Can you work these out from the drawing? Everything is in mm from the part's minimum corner. A direction names the side the tool comes from. Give positions to 0.01 mm unless a question says otherwise; leave off trailing zeros. Write each loop counter-clockwise with the first axis right and the second up, starting at its lowest first coordinate (ties: lowest second). Pieces come first, ordered by that corner, then holes. Notation, with made-up numbers: (59, 7.25) - (76, 7.25) arc R22 cw to (76, 35.25) - close; hole circle Ø6 at (7, -5.5). An arc over 180 degrees is marked (long way). Use a Markdown table: item, result.
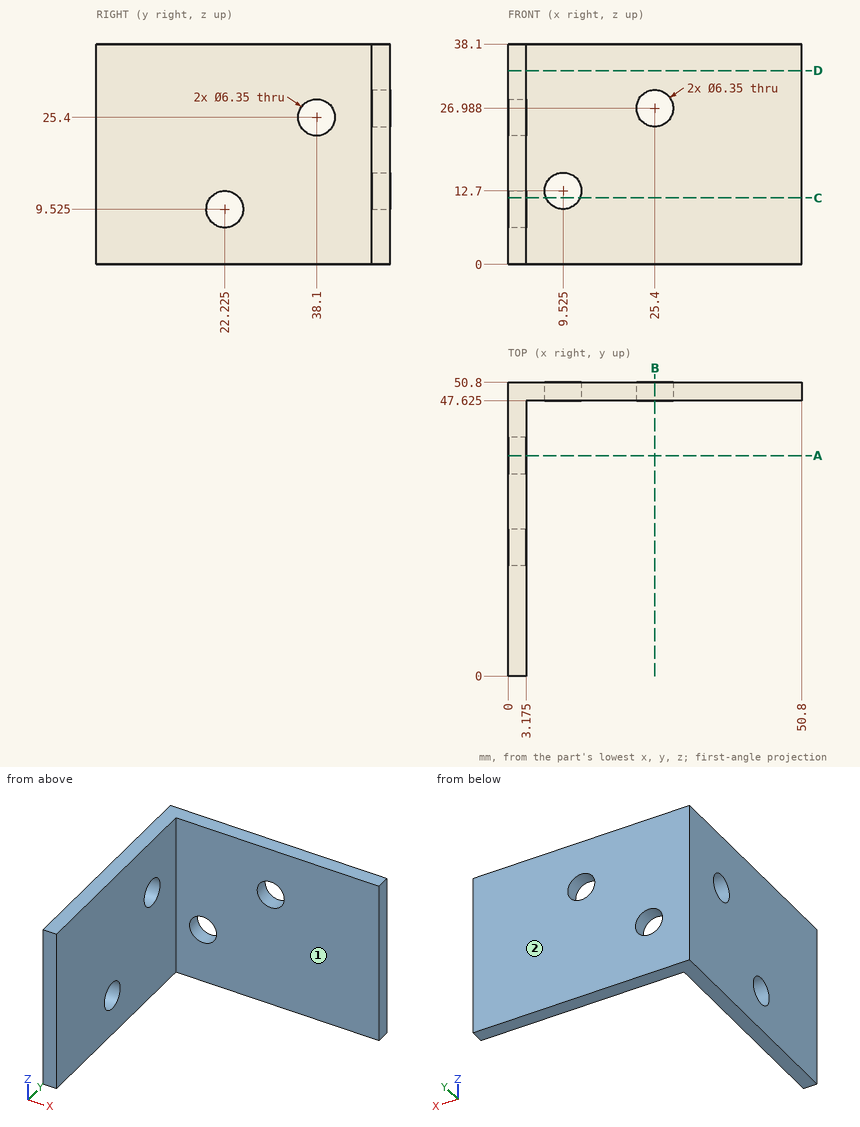
Item 1: If we section it at C-C, the plane z = 11.5: Write out the boundary of the cut face in (x, y) (1 decimal).
Values:
| item | result |
|---|---|
| outline | (0, 0) - (3.2, 0) - (3.2, 19.7) - (0, 19.7) - close; (0, 24.7) - (3.2, 24.7) - (3.2, 47.6) - (6.6, 47.6) - (6.6, 50.8) - (0, 50.8) - close; (12.5, 47.6) - (50.8, 47.6) - (50.8, 50.8) - (12.5, 50.8) - close |
Item 2: If we section it at B-B, the plane x = 25.4: Write out the boundary of the cut face in (y, z) (1 decimal).
Values:
| item | result |
|---|---|
| outline | (47.6, 0) - (50.8, 0) - (50.8, 23.8) - (47.6, 23.8) - close; (47.6, 30.2) - (50.8, 30.2) - (50.8, 38.1) - (47.6, 38.1) - close |
Item 3: If we section it at A-A, the plane y = 38.1: Write out the boundary of the cut face in (x, z) (1 decimal).
Values:
| item | result |
|---|---|
| outline | (0, 0) - (3.2, 0) - (3.2, 22.2) - (0, 22.2) - close; (0, 28.6) - (3.2, 28.6) - (3.2, 38.1) - (0, 38.1) - close |
Item 4: For the marked faces 1 and 2, which set-ups out of +Z, -Z, +X, -X, +Y, -Y let a thin tool reach every point of the face, with its end or its side?
Values:
| item | result |
|---|---|
| face 1 | +Z, -Z, +X, -Y |
| face 2 | +Z, -Z, +X, -X, +Y |
Item 5: I need wall thicknesses on line 1 along Z through (x, y) = (25.4, 49.65); line 2 along Y through (x, z) = (36.5, 24) (1 decimal); line 3 along X through (y, z) = (48.7, 12.7). Which ranges of each line are inside material? Lowest first, please. Write a range as [from, to].
Values:
| item | result |
|---|---|
| line 1 | z = [0, 23.81], [30.16, 38.1] |
| line 2 | y = [47.6, 50.8] |
| line 3 | x = [0, 6.35], [12.7, 50.8] |
Item 6: If we section it at D-D, the plane z = 33.5: Write out the boundary of the cut face in (x, y) (1 decimal).
Values:
| item | result |
|---|---|
| outline | (0, 0) - (3.2, 0) - (3.2, 47.6) - (50.8, 47.6) - (50.8, 50.8) - (0, 50.8) - close |
Item 7: Will these pins go through, and if not, where does the flat tip stop? pin 1 Ø8 at (x, z) = (9, 9.5) entering from -Y (1 decimal); pin 2 Ø10 at (y, z) = (38.1, 25.4) entering from +X (1 decimal).
Values:
| item | result |
|---|---|
| pin 1 | stops at y = 47.6 |
| pin 2 | stops at x = 3.2 |
